```python
from build123d import *

# Parameters (mm, degrees)
F0_W     = 100
F0_H     = 100
F1_DEPTH = 3
F2_DEPTH = 5
F3_D     = 2.5
F3_DEPTH = 6
F3_TIP   = 0.7510757738
F4_SIZE  = 10


with BuildPart() as f1:
    # F0 (on Top) → F1 (new body)
    with BuildSketch(Plane.XY):
        Rectangle(F0_W, F0_H)
        with BuildLine():
            Line((21.05, -22.8), (-21.05, -22.8))
            ThreePointArc((-21.05, -22.8), (-24.0374368671, -24.0374368671), (-22.8, -21.05))
            Line((-22.8, -21.05), (-22.8, 21.05))
            ThreePointArc((-22.8, 21.05), (-24.0374368671, 24.0374368671), (-21.05, 22.8))
            Line((-21.05, 22.8), (21.05, 22.8))
            ThreePointArc((21.05, 22.8), (22.8, 24.55), (24.55, 22.8))
            ThreePointArc((24.55, 22.8), (24.0374368671, 21.5625631329), (22.8, 21.05))
            Line((22.8, 21.05), (22.8, -21.05))
            ThreePointArc((22.8, -21.05), (24.0374368671, -21.5625631329), (24.55, -22.8))
            ThreePointArc((24.55, -22.8), (22.8, -24.55), (21.05, -22.8))
        make_face(mode=Mode.SUBTRACT)
        with BuildLine():
            ThreePointArc((-22.8, -21.05), (-21.5625631329, -21.5625631329), (-21.05, -22.8))
            Line((-21.05, -22.8), (21.05, -22.8))
            ThreePointArc((21.05, -22.8), (21.5625631329, -21.5625631329), (22.8, -21.05))
            Line((22.8, -21.05), (22.8, 21.05))
            ThreePointArc((22.8, 21.05), (21.5625631329, 21.5625631329), (21.05, 22.8))
            Line((21.05, 22.8), (-21.05, 22.8))
            ThreePointArc((-21.05, 22.8), (-21.5625631329, 21.5625631329), (-22.8, 21.05))
            Line((-22.8, 21.05), (-22.8, -21.05))
        make_face()
        with BuildLine():
            Line((12.65, -15.25), (-12.65, -15.25))
            ThreePointArc((-12.65, -15.25), (-17.0884776311, -17.0884776311), (-15.25, -12.65))
            Line((-15.25, -12.65), (-15.25, 12.65))
            ThreePointArc((-15.25, 12.65), (-17.0884776311, 17.0884776311), (-12.65, 15.25))
            Line((-12.65, 15.25), (12.65, 15.25))
            ThreePointArc((12.65, 15.25), (15.25, 17.85), (17.85, 15.25))
            ThreePointArc((17.85, 15.25), (17.0884776311, 13.4115223689), (15.25, 12.65))
            Line((15.25, 12.65), (15.25, -12.65))
            ThreePointArc((15.25, -12.65), (17.0884776311, -13.4115223689), (17.85, -15.25))
            ThreePointArc((17.85, -15.25), (15.25, -17.85), (12.65, -15.25))
        make_face(mode=Mode.SUBTRACT)
        with BuildLine():
            ThreePointArc((-15.25, -12.65), (-13.4115223689, -13.4115223689), (-12.65, -15.25))
            Line((-12.65, -15.25), (12.65, -15.25))
            ThreePointArc((12.65, -15.25), (13.4115223689, -13.4115223689), (15.25, -12.65))
            Line((15.25, -12.65), (15.25, 12.65))
            ThreePointArc((15.25, 12.65), (13.4115223689, 13.4115223689), (12.65, 15.25))
            Line((12.65, 15.25), (-12.65, 15.25))
            ThreePointArc((-12.65, 15.25), (-13.4115223689, 13.4115223689), (-15.25, 12.65))
            Line((-15.25, 12.65), (-15.25, -12.65))
        make_face()
    extrude(amount=-F1_DEPTH)

    # F0 (on Top) → F2 (join)
    with BuildSketch(Plane.XY):
        with BuildLine():
            Line((-15.25, -15.25), (-12.65, -15.25))
            ThreePointArc((-12.65, -15.25), (-13.4115223689, -13.4115223689), (-15.25, -12.65))
            Line((-15.25, -12.65), (-15.25, -15.25))
        make_face()
        with BuildLine():
            ThreePointArc((-15.25, -12.65), (-17.0884776311, -17.0884776311), (-12.65, -15.25))
            Line((-12.65, -15.25), (-15.25, -15.25))
            Line((-15.25, -15.25), (-15.25, -12.65))
        make_face()
        with BuildLine():
            Line((15.25, -15.25), (12.65, -15.25))
            ThreePointArc((12.65, -15.25), (15.25, -17.85), (17.85, -15.25))
            ThreePointArc((17.85, -15.25), (17.0884776311, -13.4115223689), (15.25, -12.65))
            Line((15.25, -12.65), (15.25, -15.25))
        make_face()
        with BuildLine():
            ThreePointArc((15.25, -12.65), (13.4115223689, -13.4115223689), (12.65, -15.25))
            Line((12.65, -15.25), (15.25, -15.25))
            Line((15.25, -15.25), (15.25, -12.65))
        make_face()
        with BuildLine():
            Line((-15.25, 15.25), (-15.25, 12.65))
            ThreePointArc((-15.25, 12.65), (-13.4115223689, 13.4115223689), (-12.65, 15.25))
            Line((-12.65, 15.25), (-15.25, 15.25))
        make_face()
        with BuildLine():
            ThreePointArc((-12.65, 15.25), (-17.0884776311, 17.0884776311), (-15.25, 12.65))
            Line((-15.25, 12.65), (-15.25, 15.25))
            Line((-15.25, 15.25), (-12.65, 15.25))
        make_face()
        with BuildLine():
            ThreePointArc((12.65, 15.25), (13.4115223689, 13.4115223689), (15.25, 12.65))
            Line((15.25, 12.65), (15.25, 15.25))
            Line((15.25, 15.25), (12.65, 15.25))
        make_face()
        with BuildLine():
            Line((15.25, 15.25), (15.25, 12.65))
            ThreePointArc((15.25, 12.65), (17.0884776311, 13.4115223689), (17.85, 15.25))
            ThreePointArc((17.85, 15.25), (15.25, 17.85), (12.65, 15.25))
            Line((12.65, 15.25), (15.25, 15.25))
        make_face()
    extrude(amount=-F2_DEPTH)

    # F3
    with Locations(Plane.XY):
        with Locations((-15.25, -15.25), (-15.25, 15.25), (15.25, 15.25), (15.25, -15.25)):
            Hole(F3_D / 2, depth=F3_DEPTH)
            with Locations((0, 0, -(F3_DEPTH + F3_TIP / 2))):  # 118° drill point
                Cone(0, F3_D / 2, F3_TIP, mode=Mode.SUBTRACT)

    # F4
    f4_edges = [f1.edges().sort_by_distance(p)[0] for p in [
        (-50, 50, -1.5),
        (50, 50, -1.5),
        (50, -50, -1.5),
        (-50, -50, -1.5),
    ]]
    chamfer(f4_edges, length=F4_SIZE)


solid = f1.part
```
Work out the finished part from the listing and answer in its coordinate system (mm). Give positions to 0.01 mm unless a question says otherwise; leave off trailing zeros. Loops run counter-clockwise (first coordinate to the right, second up) from the corner with the lowest first, then second, coordinate; pieces in that order, holes last. Notation, with made-up numbers: M -24,12.5 L 23,12.5 A8 cw 23,19.5 Z; hole C 12,75.25 d8. An arc over 180 degrees is marked long. One line per item, written item: value. Start each with the question number.
1. Find section B-B (x = -42.5). Give the vertices of the cut face in (y, z), and give its area (3 significant figures).
2. Determine the mould class of faces 1 (the face through (-1, -50, -1)), 2 (the face through (45, -45, -1)), 3 (the face through (-14.329, 16.095, -2.535)), 4 (the face through (-45, -45, -1)) for opening direction X: released by +X, released by -X, zero draft, split by the parting line, or undercut.
3. Find section C-C (y = 2.5). Give the vertices of the cut face in (x, z), and give its area (3 significant figures).
4. Find section A-A (z = -4.1). Give the vertices of the cut face in (x, y), and give its area (3 significant figures).
5. Find the intervals of material crossed by probe 1 along X at (y, z) = (-22.8, -1.75); probe 2 along Y at (x, z) = (15.5, -1.8), in increasing order.
6. Each of these flat-tipped pins is pushed along its axis until it touches: P1, Ø3, axis at x = -22.8, y = -22.8, coming from the -Z side; P2, Ø2, axis at x = -30, y = -24.5, coming from the -Z side. Where does it stop, or does it pass through?
Reported:
1. outline: M -47.5,-3 L 47.5,-3 L 47.5,0 L -47.5,0 Z
1. area: 285 mm²
2. face 1: zero draft
2. face 2: released by +X
2. face 3: undercut
2. face 4: released by -X
3. outline: M -50,-3 L 50,-3 L 50,0 L -50,0 Z
3. area: 300 mm²
4. outline: C -15.25,-15.25 d5.2; C -15.25,15.25 d5.2; C 15.25,-15.25 d5.2; C 15.25,15.25 d5.2; hole C -15.25,-15.25 d2.5; hole C -15.25,15.25 d2.5; hole C 15.25,-15.25 d2.5; hole C 15.25,15.25 d2.5
4. area: 65.3 mm²
5. probe 1: x = -50 to -24.55, -21.05 to 21.05, 24.55 to 50
5. probe 2: y = -50 to -16.47, -14.03 to 14.03, 16.47 to 50
6. P1: passes through
6. P2: stops at z = -3
